Geometry check sheet. Reference: the model listing, model coordinates, mm. A direction names the side the tool comes from. Coordinates: 2 decimals unless noted, no trailing zeros. Write each loop counter-clockwise with the first axis right and the second up, starting at its lowest first coordinate (ties: lowest second). Pieces come first, ordered by that corner, then holes. Notation, with made-up numbers: (77.5, 61) -> (115.5, 61) arc R9 cw to (115.5, 75) -> close; hole circle Ø7 at (47, 61.5). An arc over 180 degrees is marked (long way). One line per question, with ' | ' between items.
from build123d import *

# Parameters (mm, degrees)
SKETCH_1_W          = 118
SKETCH_1_H          = 73
SKETCH_1_R          = 1.5
EXTRUDE_1_DEPTH     = 3
EXTRUDE_2_DEPTH     = 15
SKETCH_3_W          = 3
SKETCH_3_H          = 6
EXTRUDE_3_DEPTH     = 13
SKETCH_4_W          = 3
SKETCH_4_H          = 15
EXTRUDE_4_DEPTH     = 3
SKETCH_5_W          = 3
SKETCH_5_H          = 30
EXTRUDE_5_DEPTH     = 7.5
SKETCH_7_W          = 12
SKETCH_7_H          = 24
CUT_EXTRUDE_2_DEPTH = 3
SKETCH_6_W          = 48
SKETCH_6_H          = 10.5
CUT_EXTRUDE_4_DEPTH = 3


with BuildPart() as part:
    # 草图1 → 凸台-拉伸1 (new body)
    with BuildSketch(Plane.XY):
        with Locations((26.824038132, -3.814969101)):
            Rectangle(SKETCH_1_W, SKETCH_1_H)
        with Locations((-24.175961868, 24.685030899)):
            Circle(SKETCH_1_R, mode=Mode.SUBTRACT)
        with Locations((-24.175961868, -32.314969101)):
            Circle(SKETCH_1_R, mode=Mode.SUBTRACT)
        with Locations((77.824038132, 24.685030899)):
            Circle(SKETCH_1_R, mode=Mode.SUBTRACT)
        with Locations((77.824038132, -32.314969101)):
            Circle(SKETCH_1_R, mode=Mode.SUBTRACT)
    extrude(amount=EXTRUDE_1_DEPTH)

    # 草图2 → 凸台-拉伸2 (add)
    with BuildSketch(Plane.XY.offset(3)):
        Polygon((-32.175961868, 32.685030899), (-32.175961868, 29.685030899), (-32.175961868, -37.314969101), (-32.175961868, -40.314969101), (85.824038132, -40.314969101), (85.824038132, -37.314969101), (-29.175961868, -37.314969101), (-29.175961868, 29.685030899), (85.824038132, 29.685030899), (85.824038132, 32.685030899), align=None)
    extrude(amount=EXTRUDE_2_DEPTH)

    # 草图3 → 凸台-拉伸3 (add)
    with BuildSketch(Plane.XY.offset(3)):
        Polygon((85.824038132, 3.618173266), (85.824038132, 8.685030899), (82.824038132, 8.685030899), (82.824038132, 1.685030899), (85.824038132, 1.685030899), align=None)
        with Locations((84.324038132, 26.685030899)):
            Rectangle(SKETCH_3_W, SKETCH_3_H)
        Polygon((85.824038132, -37.314969101), (85.824038132, -28.314969101), (85.2282411, -28.314969101), (82.824038132, -28.314969101), (82.824038132, -37.314969101), align=None)
    extrude(amount=EXTRUDE_3_DEPTH)

    # 草图4 → 凸台-拉伸4 (add)
    with BuildSketch(Plane.XY.offset(3)):
        with Locations((84.324038132, 16.185030899)):
            Rectangle(SKETCH_4_W, SKETCH_4_H)
    extrude(amount=EXTRUDE_4_DEPTH)

    # 草图5 → 凸台-拉伸5 (add)
    with BuildSketch(Plane.XY.offset(3)):
        with Locations((84.324038132, -13.314969101)):
            Rectangle(SKETCH_5_W, SKETCH_5_H)
    extrude(amount=EXTRUDE_5_DEPTH)

    # 草图7 → 切除-拉伸2 (cut)
    with BuildSketch(Plane.XY.offset(3)):
        Polygon((16.824038132, -35.314969101), (16.824038132, -23.314969101), (36.824038132, -23.314969101), (36.824038132, -10.314969101), (49.824038132, -10.314969101), (49.824038132, -35.314969101), align=None)
        with Locations((-23.175961868, -15.314969101)):
            Rectangle(SKETCH_7_W, SKETCH_7_H)
    extrude(amount=-CUT_EXTRUDE_2_DEPTH, mode=Mode.SUBTRACT)

    # 草图6 → 切除-拉伸4 (cut)
    with BuildSketch(Plane.XY.offset(3)):
        with Locations((1.824038132, 17.935030899)):
            Rectangle(SKETCH_6_W, SKETCH_6_H)
    extrude(amount=-CUT_EXTRUDE_4_DEPTH, mode=Mode.SUBTRACT)


solid = part.part
1. Cross-section at B-B on z = 12.5. Record the boundary of the cut face in (x, y).
Worked answers:
outline: (-32.18, -40.31) -> (85.82, -40.31) -> (85.82, -28.31) -> (82.82, -28.31) -> (82.82, -37.31) -> (-29.18, -37.31) -> (-29.18, 29.69) -> (82.82, 29.69) -> (82.82, 23.69) -> (85.82, 23.69) -> (85.82, 32.69) -> (-32.18, 32.69) -> close; (82.82, 1.69) -> (85.82, 1.69) -> (85.82, 8.69) -> (82.82, 8.69) -> close
2. Cross-section at A-A on x = -20. Record the boundary of the cut face in (y, z).
Worked answers:
outline: (-40.31, 0) -> (-27.31, 0) -> (-27.31, 3) -> (-37.31, 3) -> (-37.31, 18) -> (-40.31, 18) -> close; (-3.31, 0) -> (12.69, 0) -> (12.69, 3) -> (-3.31, 3) -> close; (23.19, 0) -> (32.69, 0) -> (32.69, 18) -> (29.69, 18) -> (29.69, 3) -> (23.19, 3) -> close
3. Cross-section at D-D on x = 32. Record the boundary of the cut face in (y, z).
Worked answers:
outline: (-40.31, 0) -> (-35.31, 0) -> (-35.31, 3) -> (-37.31, 3) -> (-37.31, 18) -> (-40.31, 18) -> close; (-23.31, 0) -> (32.69, 0) -> (32.69, 18) -> (29.69, 18) -> (29.69, 3) -> (-23.31, 3) -> close
4. Tool access check on faces 1 (the face through (16.824, -29, 2)), 2 (the face through (-29.176, -4, 9)), 3 (the face through (26, -40.315, 9)), 4 (the face through (84, -28.315, 13)). Record the directions out of +Z, -Z, +X, -X, +Y, -Y that give a thin tool (end or side, any length) a straight path to the whole face; none if there is none.
Worked answers:
face 1: +Z, -Z | face 2: +Z | face 3: +Z, -Z, +X, -X, -Y | face 4: +Z, +X
5. Cross-section at C-C on y = -7.5. Record the boundary of the cut face in (x, z), and give its area (4 significant figures).
Worked answers:
outline: (-32.18, 0) -> (-29.18, 0) -> (-29.18, 18) -> (-32.18, 18) -> close; (-17.18, 0) -> (85.82, 0) -> (85.82, 10.5) -> (82.82, 10.5) -> (82.82, 3) -> (-17.18, 3) -> close | area: 385.5 mm²
6. Material ranges on line 1 (Y direction, x = -19, z = 2); line 2 (X direction, y = -17, z = 2); line 3 (X direction, y = -35, z = 5.5), recorded low to high. Write a range as from..to.
Worked answers:
line 1: -40.31..-27.31, -3.31..12.69, 23.19..32.69 | line 2: -32.18..-29.18, -17.18..36.82, 49.82..85.82 | line 3: -32.18..-29.18, 82.82..85.82
7. Go/stop test with flat-tipped pins: P1, Ø3.5, axis at x = 77.82, y = 24.69, coming from the +Z side; P2, Ø1.5, axis at x = 84, y = 15.5, coming from the +Z side; P3, Ø1.5, axis at x = 84.5, y = -31.5, coming from the +Z side. Record where each tip stops, or that it passes through.
Worked answers:
P1: z = 3 | P2: z = 6 | P3: z = 16
8. Mould release check, pull along X, two halves, no side actions. Record for faces 5 (the face through (29, -37.315, 10)), 6 (the face through (85.824, -4, 7)), 7 (the face through (26, -3, 0)), 8 (the face through (82.824, -4, 8)): released by +X, released by -X, zero draft, split by the parting line, or undercut.
Worked answers:
face 5: undercut | face 6: released by +X | face 7: zero draft | face 8: undercut
